Check sheet for the modelled part. Datum: model origin and axes. Units: mm. Give positions to 0.01 mm unless a question says otherwise; leave off trailing zeros. Loops run counter-clockwise (first coordinate to the right, second up) from the corner with the lowest first, then second, coordinate; pieces in that order, holes last. Notation, with made-up numbers: (65.5, -37.5) -> (122.5, -37.5) arc R10 ccw to (122.5, -25.5) -> close; hole circle Ø11 at (84.5, 6). An arc over 180 degrees is marked (long way). Write each question's results on one line, items separated by ' | '. Start each with the question number.
1. Cross-section at B-B on x = 14. Record the boundary of the cut face in (y, z).
2. Material ranges on L1, parallel to X at y = 0.85, z = -35.5; L2, parallel to Z at x = 14, y = 1.3; L3, parallel to X at y = 1.1, z = 0 (3 decimals), recorded low to high. Write a range as from..to.
3. Cross-section at C-C on y = 0.8. Record the boundary of the cut face in (x, z) (3 decimals), and give its area (3 significant figures).
4. Cross-section at D-D on z = 0. Record the boundary of the cut face in (x, y) (3 decimals).
5. Cross-section at A-A on z = -35.5. Record the boundary of the cut face in (x, y), and give its area (3 significant figures).
6. Gauge pin test, flat ends, axial feed: pin 1 Ø0.8 at (y, z) = (1, -2) entering from -X (3 decimals); pin 2 Ø1 at (x, z) = (-13.5, -47.5) entering from -Y; pin 3 Ø0.8 at (y, z) = (0.5, 13.5) entering from +X (3 decimals); pin 4 Ø3 at (x, z) = (-14, -35.5) entering from -Y. Record the tip position at first contact, or that the pin passes through.
from build123d import *

# Parameters (mm, degrees)
BOSS_EXTRUDE1_DEPTH            = 1.6
CHAMFER1_SIZE                  = 0.45
CHAMFER1_SIZE2                 = 0.779422863
FILLET1_R                      = 1
CUT_EXTRUDE1_DEPTH             = 2.6
F_3_2_3_2_DIAMETER_HOLE1_D     = 3.2
F_3_2_3_2_DIAMETER_HOLE1_DEPTH = 1.6
F_3_2_3_2_DIAMETER_HOLE1_TIP   = 0.96137699


with BuildPart() as part:
    # Sketch1 → Boss-Extrude1 (new body)
    with BuildSketch(Plane(origin=(0, 0, 0), x_dir=(1, 0, 0), z_dir=(0, 1, 0))):
        Polygon((-7.425, 15.5), (-18, 15.5), (-18, 55.5), (18, 55.5), (18, 15.5), (7.425, 15.5), (7.425, -15.5), (-7.425, -15.5), align=None)
    extrude(amount=BOSS_EXTRUDE1_DEPTH)

    # Chamfer1
    chamfer1_edges = [part.edges().sort_by_distance(p)[0] for p in [
        (0, 1.6, 15.5),
        (0, 0, 15.5),
    ]]
    chamfer1_side = [part.faces().sort_by_distance(p)[0] for p in [
        (0, 0.8, 15.5),
    ]]
    chamfer(chamfer1_edges, length=CHAMFER1_SIZE, length2=CHAMFER1_SIZE2, reference=chamfer1_side[0])

    # Fillet1
    fillet1_edges = [part.edges().sort_by_distance(p)[0] for p in [
        (-7.425, 0.8, -15.5),
        (-18, 0.8, -15.5),
        (-18, 0.8, -55.5),
        (18, 0.8, -55.5),
        (18, 0.8, -15.5),
        (7.425, 0.8, -15.5),
    ]]
    fillet(fillet1_edges, radius=FILLET1_R)

    # Sketch2 → Cut-Extrude1 (cut, through all)
    with BuildSketch(Plane(origin=(0, 1.6, 0), x_dir=(1, 0, 0), z_dir=(0, 1, 0))):
        with BuildLine():
            Line((-1.595, -10.3), (-1.595, -15.5))
            Line((-1.595, -15.5), (0.805, -15.5))
            Line((0.805, -15.5), (0.805, -10.3))
            ThreePointArc((0.805, -10.3), (-0.395, -9.1), (-1.595, -10.3))
        make_face()
    extrude(amount=-CUT_EXTRUDE1_DEPTH, mode=Mode.SUBTRACT)

    # Ø3.2 (3.2) Diameter Hole1
    with Locations(Plane(origin=(-14, 1.6, -35.5), x_dir=(0, 0, 1), z_dir=(0, 1, 0))):
        with Locations((0, 0), (0, 28)):
            Hole(F_3_2_3_2_DIAMETER_HOLE1_D / 2, depth=F_3_2_3_2_DIAMETER_HOLE1_DEPTH)
            with Locations((0, 0, -(F_3_2_3_2_DIAMETER_HOLE1_DEPTH + F_3_2_3_2_DIAMETER_HOLE1_TIP / 2))):  # 118° drill point
                Cone(0, F_3_2_3_2_DIAMETER_HOLE1_D / 2, F_3_2_3_2_DIAMETER_HOLE1_TIP, mode=Mode.SUBTRACT)


solid = part.part
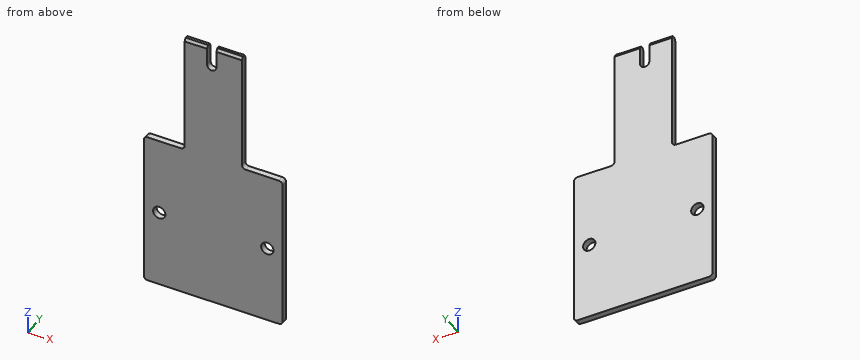
Geometry says:
1) outline: (0, -55.5) -> (1.6, -55.5) -> (1.6, -37.1) -> (0, -37.1) -> close; (0, -33.9) -> (1.6, -33.9) -> (1.6, -15.5) -> (0, -15.5) -> close
2) L1: -18..-15.6, -12.4..12.4, 15.6..18 | L2: -55.5..-37.1, -33.9..-15.5 | L3: -7.425..7.425
3) outline: (-18, -54.5) arc R1 ccw to (-17, -55.5) -> (17, -55.5) arc R1 ccw to (18, -54.5) -> (18, -16.5) arc R1 ccw to (17, -15.5) -> (8.425, -15.5) arc R1 cw to (7.425, -14.5) -> (7.425, 15.5) -> (0.805, 15.5) -> (0.805, 10.3) arc R1.2 cw to (-1.595, 10.3) -> (-1.595, 15.5) -> (-7.425, 15.5) -> (-7.425, -14.5) arc R1 cw to (-8.425, -15.5) -> (-17, -15.5) arc R1 ccw to (-18, -16.5) -> close; hole circle Ø3.2 at (-14, -35.5); hole circle Ø3.2 at (14, -35.5) | area: 1,870 mm^2
4) outline: (-7.425, 0) -> (7.425, 0) -> (7.425, 1.6) -> (-7.425, 1.6) -> close
5) outline: (-18, 0) -> (-15.6, 0) -> (-15.6, 1.6) -> (-18, 1.6) -> close; (-12.4, 0) -> (12.4, 0) -> (12.4, 1.6) -> (-12.4, 1.6) -> close; (15.6, 0) -> (18, 0) -> (18, 1.6) -> (15.6, 1.6) -> close | area: 47.4 mm^2
6) pin 1: x = -7.425 | pin 2: y = 0 | pin 3: x = 7.425 | pin 4: through
